For this review, take the finished solid that the model builds, in its own axes (mm). A direction names the side the tool comes from. Give positions to 0.01 mm unless a question says otherwise; leave off trailing zeros. Loops run counter-clockwise (first coordinate to the right, second up) from the corner with the lowest first, then second, coordinate; pieces in that order, holes last. Notation, with made-up numbers: M -32,64 L 14,64 A31 cw 14,93 Z; hole C -20,89.5 d9. An arc over 180 degrees is marked long. Use CSV: the item, a comma, the result in double quotes. Start each with the question number.
1. Tool access review of faces 1 (the face through (-13.05, -7.4, -0.49)), 2 (the face through (100, 0, 15)), 3 (the face through (179.167, 7.35, -27.535)), 4 (the face through (239.662, -26.81, 0.42)): name each direction out of +Z, -Z, +X, -X, +Y, -Y from which nothing blocks a thin tool from reaching the whole face with its end or side.
2. Take a section at A-A, the plane x = 339. Write out the cut boundary in (y, z).
3. Take a section at B-B, the plane x = 0. Write out the cut boundary in (y, z).
4. To check wall thickness, follow line 1 (Y direction, x = 175, z = -2); line 2 (Y direction, x = -1, z = -29.5); line 3 (X direction, y = 18, z = -6). State the ranges of each line that lie inside material, in increasing order. Write a range as [from, to].
5. Insertion check: P1, Ø8.5, axis at x = -1.5, z = -12.5, coming from the -Y side; P2, Ø6.5, axis at x = 188.54, y = 17.08, coming from the +Z side; P3, Ø8, axis at x = 260, z = 5.5, coming from the +Y side. Each pin has a flat end and moves straight along its axis. Give the tip position at first contact, or say it passes through.
6. The part is to be moulded in two halves that separate along X. For faces 5 (the face through (274.541, 5.966, 0.21)), 6 (the face through (366, 24, 35)), say which applies: pulls with the +X half, pulls with the -X half, needs draft (parallel to the pull), parting line crosses it, or undercut.
from build123d import *
from build123d.topology import SkipClean

# Parameters (mm, degrees)
LEFT_ARM_DEPTH                = 15
SKETCH2_R                     = 27.5
LEFT_BOSS_DEPTH               = 35
LEFT_HEX_DEPTH                = 265.244205
LEFT_HEX_DEPTH_BACK           = 265.244205
SKETCH3_R                     = 70
CENTRE_BOSS_DEPTH             = 30
SKETCH5_W                     = 30
SKETCH5_H                     = 40
RIGHT_ARM_DEPTH               = 175
SKETCH7_R                     = 50
RIGHT_BOSS_DEPTH              = 35
SKETCH8_R                     = 30
RIGHT_BOSS_HOLE_DEPTH         = 412.395178
SKETCH9_R                     = 40
CENTRE_HOLE_DEPTH             = 411.573979
SKETCH10_R                    = 27.5
CENTRE_BLOB_DEPTH             = 30
CENTRE_BEAM_REACH             = 243.419
SKETCH11_W                    = 10
SKETCH11_H                    = 30
CENTRE_BEAM_DIRECTION_2_REACH = 243.419
SKETCH12_R                    = 20
CUT_EXTRUDE4_DEPTH            = 5
M6X1_0_TAPPED_HOLE1_D         = 5
CIRPATTERN1_COUNT             = 6
CUT_OUT_DEPTH                 = 10
FILLET1_R                     = 10
FILLET1_OF_MIRROR2_R          = 10
KEYWAY_DEPTH                  = 407.904156


with BuildPart() as part:
    # Sketch1 → LEFT_ARM (new, symmetric)
    with BuildSketch(Plane.XY):
        with BuildLine():
            Line((-6.678571, 26.676707), (158, 67.904344))
            ThreePointArc((158, 67.904344), (245, 0), (158, -67.904344))
            Line((158, -67.904344), (-6.678571, -26.676707))
            ThreePointArc((-6.678571, -26.676707), (-27.5, 0), (-6.678571, 26.676707))
        make_face()
    extrude(amount=LEFT_ARM_DEPTH, both=True)

    # Sketch2 → LEFT_Boss (add, symmetric)
    with SkipClean():  # the faces are left unmerged after this step: merging them gives an invalid solid
        with BuildSketch(Plane.XY):
            Circle(SKETCH2_R)
        extrude(amount=LEFT_BOSS_DEPTH, both=True)

    # Sketch4 → LEFT_Hex (cut, two sides: drawn at the far end of the back side and taken through both)
    with SkipClean():  # the faces are left unmerged after this step: merging them gives an invalid solid
        with BuildSketch(Plane.XY.offset(35).offset(-LEFT_HEX_DEPTH_BACK)):
            Polygon((17.320508, 0), (8.660254, 15), (-8.660254, 15), (-17.320508, 0), (-8.660254, -15), (8.660254, -15), align=None)
        extrude(amount=LEFT_HEX_DEPTH + LEFT_HEX_DEPTH_BACK, mode=Mode.SUBTRACT)

    # Sketch3 → CENTRE_Boss (add, symmetric)
    with BuildSketch(Plane.XY):
        with Locations((175, 0)):
            Circle(SKETCH3_R)
    extrude(amount=CENTRE_BOSS_DEPTH, both=True)

    # Sketch5 → RIGHT_ARM (add)
    with BuildSketch(Plane(origin=(163.277223, 43.75, 0), x_dir=(0, 0, -1), z_dir=(0.9659258262890681, 0.25881904510252135, 0))):
        with Locations((0, -45.293333)):
            Rectangle(SKETCH5_W, SKETCH5_H)
    extrude(amount=RIGHT_ARM_DEPTH)

    # Sketch7 → RIGHT_Boss (add, symmetric)
    with BuildSketch(Plane.XY):
        with Locations((344.03702, 45.293333)):
            Circle(SKETCH7_R)
    extrude(amount=RIGHT_BOSS_DEPTH, both=True)

    # Sketch8 → RIGHT_Boss_Hole (cut, through all)
    with BuildSketch(Plane.XY.offset(35)):
        with Locations((344.03702, 45.293333)):
            Circle(SKETCH8_R)
    extrude(amount=-RIGHT_BOSS_HOLE_DEPTH, mode=Mode.SUBTRACT)

    # Sketch9 → CENTRE_Hole (cut, through all)
    with BuildSketch(Plane.XY.offset(30)):
        with Locations((175, 0)):
            Circle(SKETCH9_R)
    extrude(amount=-CENTRE_HOLE_DEPTH, mode=Mode.SUBTRACT)

    # Sketch10 → CENTRE_Blob (add, symmetric)
    with BuildSketch(Plane.XY):
        with Locations((199.148146, 6.470476)):
            Circle(SKETCH10_R)
    extrude(amount=CENTRE_BLOB_DEPTH, both=True)

    # Sketch11 → CENTRE_Beam (add, up to next)
    with BuildSketch(Plane(origin=(175, 0, 0), x_dir=(0, 0, -1), z_dir=(1, 0, 0)), mode=Mode.PRIVATE) as centre_beam_sk1:
        Rectangle(SKETCH11_W, SKETCH11_H)
    centre_beam_tool1 = extrude(centre_beam_sk1.sketch, amount=CENTRE_BEAM_REACH, mode=Mode.PRIVATE) - part.part
    add(centre_beam_tool1.solids().sort_by_distance((175, 0, 0))[0])

    # Sketch11 → CENTRE_Beam direction 2 (add, up to next)
    with BuildSketch(Plane(origin=(175, 0, 0), x_dir=(0, 0, -1), z_dir=(1, 0, 0)), mode=Mode.PRIVATE) as centre_beam_direction_2_sk1:
        Rectangle(SKETCH11_W, SKETCH11_H)
    centre_beam_direction_2_tool1 = extrude(centre_beam_direction_2_sk1.sketch, amount=-CENTRE_BEAM_DIRECTION_2_REACH, mode=Mode.PRIVATE) - part.part
    add(centre_beam_direction_2_tool1.solids().sort_by_distance((175, 0, 0))[0])

    # Sketch12 → Cut-Extrude4 (cut)
    with BuildSketch(Plane.XY.offset(30)):
        with Locations((199.148146, 6.470476)):
            Circle(SKETCH12_R)
    cut_extrude4 = extrude(amount=-CUT_EXTRUDE4_DEPTH, mode=Mode.SUBTRACT)

    # M6x1.0 Tapped Hole1 (through all)
    with Locations(Plane.XY.offset(25)):
        with Locations((184.659258, 2.58819)):
            m6x1_0_tapped_hole1 = Hole(M6X1_0_TAPPED_HOLE1_D / 2)

    # CirPattern1: M6x1.0 Tapped Hole1 ×6 about axis
    cirpattern1_axis = Axis((199.148146, 6.470476, 0), (0, 0, 1))
    for i in range(1, CIRPATTERN1_COUNT):
        add(m6x1_0_tapped_hole1.rotate(cirpattern1_axis, i * 360 / CIRPATTERN1_COUNT), mode=Mode.SUBTRACT)

    # Mirror1: Cut-Extrude4 across plane
    add(cut_extrude4.mirror(Plane.XY), mode=Mode.SUBTRACT)

    # Sketch15 → Cut_OUT (cut)
    with BuildSketch(Plane.XY.offset(15)):
        with BuildLine():
            Line((109.097712, 45.352932), (27.923319, 25.030746))
            ThreePointArc((27.923319, 25.030746), (37.5, 0), (27.923319, -25.030746))
            Line((27.923319, -25.030746), (109.097712, -45.352932))
            ThreePointArc((109.097712, -45.352932), (95, 0), (109.097712, 45.352932))
        make_face()
    cut_out = extrude(amount=-CUT_OUT_DEPTH, mode=Mode.SUBTRACT)

    # Fillet1
    fillet1_edges = [part.edges().sort_by_distance(p)[0] for p in [
        (27.923319, -25.030746, 10),
        (27.923319, 25.030746, 10),
        (109.097712, 45.352932, 10),
        (109.097712, -45.352932, 10),
    ]]
    fillet(fillet1_edges, radius=FILLET1_R)

    # Mirror2: Cut_OUT across plane
    with SkipClean():  # the faces are left unmerged after this step: merging them gives an invalid solid
        add(cut_out.mirror(Plane.XY), mode=Mode.SUBTRACT)

    # Fillet1 of Mirror2
    fillet1_of_mirror2_edges = [part.edges().sort_by_distance(p)[0] for p in [
        (27.923319, -25.030746, -10),
        (27.923319, 25.030746, -10),
        (109.097712, 45.352932, -10),
        (109.097712, -45.352932, -10),
    ]]
    fillet(fillet1_of_mirror2_edges, radius=FILLET1_OF_MIRROR2_R)

    # Sketch16 → KEYWAY (cut, symmetric)
    with SkipClean():  # the faces are left unmerged after this step: merging them gives an invalid solid
        with BuildSketch(Plane.XY):
            Polygon((346.366391, 36.6), (341.707648, 53.986665), (308.4798, 45.08329), (313.138543, 27.696625), align=None)
        keyway = extrude(amount=KEYWAY_DEPTH, both=True, mode=Mode.SUBTRACT)

    # Mirror3: KEYWAY across plane
    with SkipClean():  # the faces are left unmerged after this step: merging them gives an invalid solid
        add(keyway.mirror(Plane(origin=(332.314242, 89.043333, 0), x_dir=(0, 0, 1), z_dir=(0.9659258262890681, 0.25881904510252135, 0))), mode=Mode.SUBTRACT)


solid = part.part
Result set:
1,face 1,"+Z, -Z"
1,face 2,"+Z"
1,face 3,"-Z"
1,face 4,"none"
2,outline,"M -4.45,-35 L 15.72,-35 L 15.72,35 L -4.45,35 Z; M 74.87,-35 L 95.04,-35 L 95.04,35 L 74.87,35 Z"
3,outline,"M -28.35,-15 L -27.5,-15 L -27.5,-35 L -15,-35 L -15,35 L -27.5,35 L -27.5,15 L -28.35,15 Z; M 15,-35 L 27.5,-35 L 27.5,-15 L 28.35,-15 L 28.35,15 L 27.5,15 L 27.5,35 L 15,35 Z"
4,line 1,"[-70, -40], [-15, 19.63], [40, 70]"
4,line 2,"[-27.48, -15], [15, 27.48]"
4,line 3,"[-20.79, 33.7], [97.05, 139.28], [174.18, 186.22], [190.86, 331.58], [356.49, 385.93]"
5,P1,"y = -29.04"
5,P2,"z = 25"
5,P3,"y = 44.55"
6,face 5,"undercut"
6,face 6,"needs draft"
